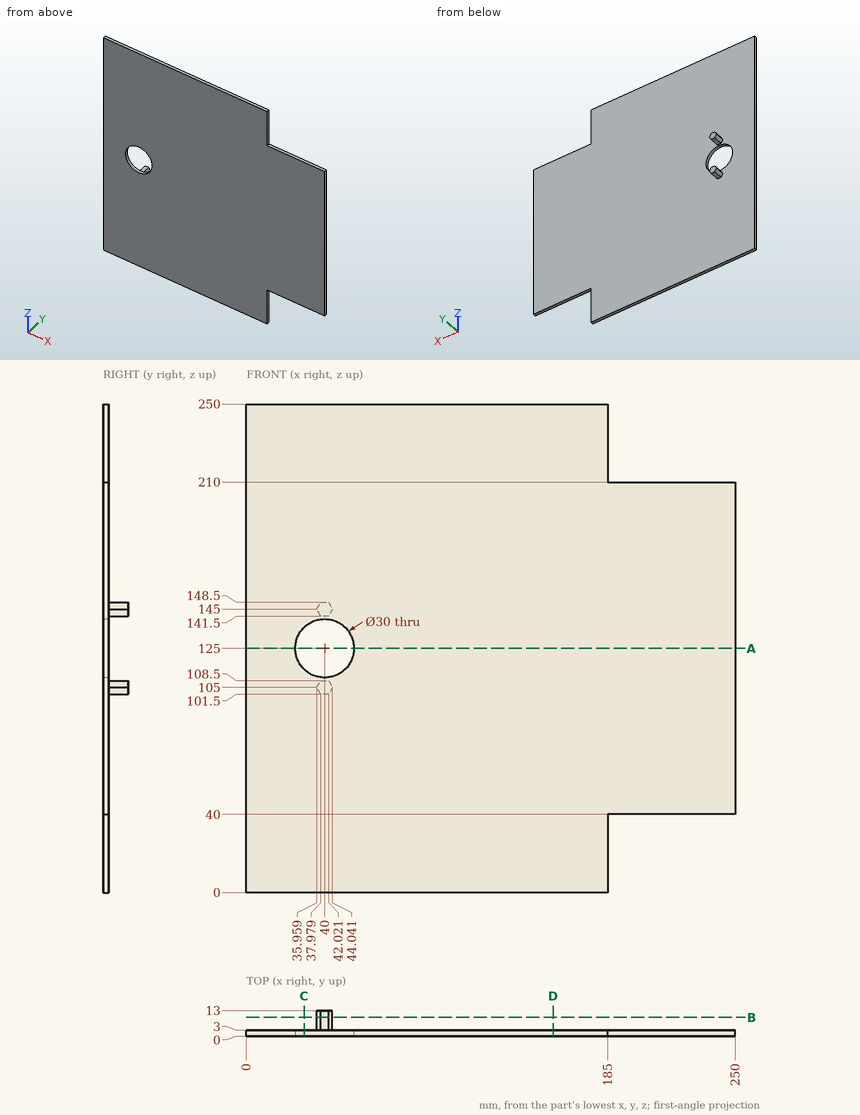
Source: three-view drawing plus pictorial views. Frame: mm from the lowest corner of the part. Give positions to 0.01 mm unless a question says otherwise; leave off trailing zeros. Write each loop counter-clockwise with the first axis right and the second up, starting at its lowest first coordinate (ties: lowest second). Pieces come first, ordered by that corner, then holes.
(1) Cut plane C-C, the plane x = 29.5. Return loops of the section in (y, z).
(2) First-contact query: P1, Ø4.5, axis at x = 40.5, y = 10, coming from the +Z side; P2, Ø4.5, axis at x = 40.5, y = 9, coming from the -Z side; P3, Ø6, axis at x = 150, y = 8, coming from the -Z side; P4, Ø1.5, axis at x = 224, y = 1.5, coming from the -Z side. Flat tips, straight axial feed; report the tip coordinate or a pass-through.
(3) Cut plane A-A, the plane z = 125. Return loops of the section in (x, y), then the cut area to 3 significant figures.
(4) Ray query, line 1 (X direction, y = 0.7, z = 125); line 2 (Y direction, x = 98.5, z = 48). Return the intervals inside material, ascending.
(5) Cut plane D-D, the plane x = 157. Return loops of the section in (y, z), then the cut area to 3 significant figures.
(6) Cut plane B-B, the plane y = 9.5. Return loops of the section in (x, z).
Values follow:
1. outline: (0, 0) - (3, 0) - (3, 114.29) - (0, 114.29) - close; (0, 135.71) - (3, 135.71) - (3, 250) - (0, 250) - close
2. P1: stops at z = 148.5
2. P2: stops at z = 101.5
2. P3: passes through
2. P4: stops at z = 40
3. outline: (0, 0) - (25, 0) - (25, 3) - (0, 3) - close; (55, 0) - (250, 0) - (250, 3) - (55, 3) - close
3. area: 660 mm2
4. line 1: x = 0 to 25, 55 to 250
4. line 2: y = 0 to 3
5. outline: (0, 0) - (3, 0) - (3, 250) - (0, 250) - close
5. area: 750 mm2
6. outline: (35.96, 105) - (37.98, 101.5) - (42.02, 101.5) - (44.04, 105) - (42.02, 108.5) - (37.98, 108.5) - close; (35.96, 145) - (37.98, 141.5) - (42.02, 141.5) - (44.04, 145) - (42.02, 148.5) - (37.98, 148.5) - close
